Here's how the part is built. I have some questions about the finished solid (model axes, mm). A direction names the side the tool comes from. Coordinates: 2 decimals unless noted, no trailing zeros. Write each loop counter-clockwise with the first axis right and the second up, starting at its lowest first coordinate (ties: lowest second). Pieces come first, ordered by that corner, then holes.
```python
from build123d import *

# Parameters (mm, degrees)
F0_W     = 50.8
F0_H     = 50.8
F1_DEPTH = 7.62
F2_W     = 40.64
F2_H     = 40.64
F3_DEPTH = 25.4
F4_R     = 7.62
F6_R     = 4.445


with BuildPart() as f1:
    # F0 (on Top) → F1 (new body)
    with BuildSketch(Plane.XY):
        Rectangle(F0_W, F0_H)
    extrude(amount=F1_DEPTH)

    # F2 (on face) → F3 (join)
    with BuildSketch(Plane.XY.offset(7.62)):
        Rectangle(F2_W, F2_H)
    extrude(amount=F3_DEPTH)

    # F4 (on face) → F7 section 0
    with BuildSketch(Plane.XY.offset(33.02)):
        Circle(F4_R)
    # F6 (on offset) → F7 section 1
    with BuildSketch(Plane.XY.offset(38.1)):
        Circle(F6_R)
    loft()

    # F9 (on offset) → F10 (revolve)
    with BuildSketch(Plane.YZ):
        with BuildLine():
            Line((0, 37.4538087019), (0, 36.551290824))
            ThreePointArc((0, 36.551290824), (26.302517878, 62.8538087019), (0, 89.1563265799))
            Line((0, 89.1563265799), (0, 88.2538087019))
            Line((0, 88.2538087019), (0, 37.4538087019))
        make_face()
    revolve(axis=Axis((0, 0, 62.8538087019), (0, 0, -1)))


solid = f1.part
```
1) Imagine slicing it at B-B on x = 0. Please give me the cut outline in (y, z), then the cut area to 3 significant figures.
Values follow:
outline: (-25.4, 0) - (25.4, 0) - (25.4, 7.62) - (20.32, 7.62) - (20.32, 33.02) - (7.62, 33.02) - (5.1, 37.05) arc R26.3 ccw (long way) to (-5.1, 37.05) - (-7.62, 33.02) - (-20.32, 33.02) - (-20.32, 7.62) - (-25.4, 7.62) - close
area: 3,640 mm2
2) Imagine slicing it at C-C on z = 18. Please give me the cut outline in (x, y).
Values follow:
outline: (-20.32, -20.32) - (20.32, -20.32) - (20.32, 20.32) - (-20.32, 20.32) - close
3) Imagine slicing it at D-D on z = 54. Please give me the cut outline in (x, y), then the cut area to 3 significant figures.
Values follow:
outline: circle Ø49.54 at (0, 0)
area: 1,930 mm2
4) I need wall thicknesses on probe 1 along X at (y, z) = (-10.5, 14); probe 2 along Z at (x, y) = (12.5, 10.5); probe 3 along Z at (x, y) = (-5.5, -14.5). Which ranges of each line are inside material? Lowest first, please.
Values follow:
probe 1: x = -20.32 to 20.32
probe 2: z = 0 to 33.02, 42.23 to 83.48
probe 3: z = 0 to 33.02, 41.61 to 84.1
5) We'd pull the mould along Z, two halves only. Please class faces 1 (the face through (0, 25.4, 4)), 2 (the face through (0, 0, 0)), 3 (the face through (0, -20.32, 20)): pulls with the +Z half, pulls with the -Z half, needs draft (parallel to the pull), parting line crosses it, or undercut.
Values follow:
face 1: needs draft
face 2: pulls with the -Z half
face 3: undercut
6) Imagine slicing it at A-A on y = 11.5. Please give me the cut outline in (x, z).
Values follow:
outline: (-25.4, 0) - (25.4, 0) - (25.4, 7.62) - (20.32, 7.62) - (20.32, 33.02) - (-20.32, 33.02) - (-20.32, 7.62) - (-25.4, 7.62) - close; circle Ø47.31 at (0, 62.85)
7) On a 3-axis mill with a long thin cutter (end or side, diameter ignored), from which of +Z, -Z, +X, -X, +Y, -Y can I reach the whole of each face in a straight line? I mean faces 4 (the face through (0, -25.4, 4)), 5 (the face through (20.32, 0, 20)), 6 (the face through (25.4, 0, 4)), 7 (the face through (9, 0, 33.02)). Say none if no direction works.
Values follow:
face 4: -Z, +X, -X, -Y
face 5: +X, +Y, -Y
face 6: -Z, +X, +Y, -Y
face 7: none
8) Will these pins go through, and if not, where does the flat tip stop? pin 1 (12.5 mm diameter, centred on y = -3.5, z = 25.5, fed in from -X); pin 2 (1.5 mm diameter, centred on x = -5.5, z = 41, fed in from +Y); pin 3 (1 mm diameter, centred on x = -1.5, z = 40.5, fed in from -Y); pin 4 (6 mm diameter, centred on y = -3, z = 63, fed in from -X).
Values follow:
pin 1: stops at x = -20.32
pin 2: stops at y = 14.74
pin 3: stops at y = -14.56
pin 4: stops at x = -26.3
